```python
from build123d import *

# Parameters (mm, degrees)
ESQUISSE6_W             = 6
ESQUISSE6_H             = 6
BOSS_EXTRU_2_DEPTH      = 20.7
ENL_V_MAT_EXTRU_1_DEPTH = 10


with BuildPart() as part:
    # Esquisse2 → Révolution1 (revolve)
    with BuildSketch(Plane(origin=(0, 0, 0), x_dir=(0, 0, -1), z_dir=(1, 0, 0))):
        Polygon((0, 0), (33.95, 0), (33.95, 3), (5, 3), (5, 5), (0, 5), align=None)
    revolve(axis=Axis((0, 0, 0), (0, 0, -1)))

    # Esquisse6 → Boss.-Extru.2 (add)
    with BuildSketch(Plane(origin=(0, 0, -5), x_dir=(-1, 0, 0), z_dir=(0, 0, -1))):
        Rectangle(ESQUISSE6_W, ESQUISSE6_H)
    extrude(amount=BOSS_EXTRU_2_DEPTH)

    # Esquisse4 → Enlèv. mat.-Extru.1 (cut)
    with BuildSketch(Plane(origin=(0, 0, -33.95), x_dir=(-1, 0, 0), z_dir=(0, 0, -1))):
        with BuildLine():
            Line((-1.204159458, 1.2), (1.204159458, 1.2))
            ThreePointArc((1.204159458, 1.2), (0, -1.7), (-1.204159458, 1.2))
        make_face()
    extrude(amount=-ENL_V_MAT_EXTRU_1_DEPTH, mode=Mode.SUBTRACT)


solid = part.part
```
Part model, mm, in its own coordinate system. A direction names the side the tool comes from. Round coordinates to 2 decimals unless told otherwise and drop trailing zeros. Write each loop counter-clockwise with the first axis right and the second up, starting at its lowest first coordinate (ties: lowest second). Pieces come first, ordered by that corner, then holes. Notation, with made-up numbers: M 45,12 L 73,12 A22 ccw 73,34 Z; hole C 46.5,87 d6. An arc over 180 degrees is marked long. Answer as CSV lines item,"result". Start each with the question number.
1) Drop flat-ended pins along their axis: pin 1 (4 mm diameter, centred on x = 0, y = 0, fed in from +Z); pin 2 (3 mm diameter, centred on y = 2, z = -26, fed in from +X); pin 3 (3 mm diameter, centred on x = -0.5, z = -16.5, fed in from -Y); pin 4 (6 mm diameter, centred on x = -3.5, z = -17, fed in from +Y). Give the stop position or say it passes through.
2) Band-saw the part on B-B (y = 2). List the corners of the cut face in (x, z), then the cut area to 3 significant figures.
3) Band-saw the part on A-A (z = -24.5). List the corners of the cut face in (x, y).
4) Band-saw the part on D-D (z = -1.5). List the corners of the cut face in (x, y).
5) Band-saw the part on C-C (x = 2.25). List the corners of the cut face in (y, z).
6) Which spindle directions (+Z, -Z, +X, -X, +Y, -Y) get a long thin tool onto all of the face, cutting with end or side? Do faces 1 (the face through (3, 0, -15)), 2 (the face through (0, 3, -15)), 3 (the face through (-3, 0, -15)). Say none if no direction does.
7) Drill centre lines: L1, parallel to Y at x = 0, z = -27; L2, parallel to X at y = 0, z = -30.75; L3, parallel to X at y = -0.5, z = -9.5. Where is each one in solid material? Low to high.
8) Mould opens along X. For faces 4 (the face through (-2.4, -2.4, -25.7)), 5 (the face through (-0.06, -1.7, -29.02)), 6 (the face through (0, -3, -30)) say: +X half, -X half, draft (parallel to the pull), parting line (faces both ways), or undercut.
Worked out:
1,pin 1,"z = 0"
1,pin 2,"x = 3"
1,pin 3,"y = -3"
1,pin 4,"y = 3"
2,outline,"M -4.58,-5 L -3,-5 L -3,-25.7 L -2.24,-25.7 L -2.24,-33.95 L 2.24,-33.95 L 2.24,-25.7 L 3,-25.7 L 3,-5 L 4.58,-5 L 4.58,0 L -4.58,0 Z"
2,area,"207 mm²"
3,outline,"M -3,-3 L 3,-3 L 3,3 L -3,3 Z; hole M -1.2,1.2 A1.7 ccw long 1.2,1.2 Z"
4,outline,"C 0,0 d10"
5,outline,"M -4.47,-5 L -3,-5 L -3,-25.7 L -1.98,-25.7 L -1.98,-33.95 L 1.98,-33.95 L 1.98,-25.7 L 3,-25.7 L 3,-5 L 4.47,-5 L 4.47,0 L -4.47,0 Z"
6,face 1,"-Z, +X, +Y, -Y"
6,face 2,"-Z, +X, -X, +Y"
6,face 3,"-Z, -X, +Y, -Y"
7,L1,"-3 to -1.7, 1.2 to 3"
7,L2,"-3 to -1.7, 1.7 to 3"
7,L3,"-3 to 3"
8,face 4,"draft"
8,face 5,"undercut"
8,face 6,"parting line"
